from build123d import *

# Parameters (mm, degrees)
SKETCH1_W           = 21
SKETCH1_H           = 30
SKETCH1_R           = 1.75
BOSS_EXTRUDE1_DEPTH = 4
SKETCH2_W           = 21
SKETCH2_H           = 6.5
CUT_EXTRUDE1_DEPTH  = 1
SKETCH3_W           = 1
SKETCH3_H           = 6.5
BOSS_EXTRUDE2_DEPTH = 1
CHAMFER1_SIZE       = 0.5
CHAMFER2_SIZE       = 0.5


with BuildPart() as part:
    # Sketch1 → Boss-Extrude1 (new body)
    with BuildSketch(Plane.XY):
        with Locations((10.5, 15)):
            Rectangle(SKETCH1_W, SKETCH1_H)
        with Locations((4, 4)):
            Circle(SKETCH1_R, mode=Mode.SUBTRACT)
        with Locations((17, 4)):
            Circle(SKETCH1_R, mode=Mode.SUBTRACT)
        with Locations((17, 26)):
            Circle(SKETCH1_R, mode=Mode.SUBTRACT)
        with Locations((4, 26)):
            Circle(SKETCH1_R, mode=Mode.SUBTRACT)
    extrude(amount=BOSS_EXTRUDE1_DEPTH)

    # Sketch2 → Cut-Extrude1 (cut)
    with BuildSketch(Plane.XY.offset(4)):
        with Locations((10.5, 15)):
            Rectangle(SKETCH2_W, SKETCH2_H)
    extrude(amount=-CUT_EXTRUDE1_DEPTH, mode=Mode.SUBTRACT)

    # Sketch3 → Boss-Extrude2 (add)
    with BuildSketch(Plane.XY.offset(3)):
        with Locations((0.5, 15)):
            Rectangle(SKETCH3_W, SKETCH3_H)
        with Locations((2.5, 15)):
            Rectangle(SKETCH3_W, SKETCH3_H)
        with Locations((4.5, 15)):
            Rectangle(SKETCH3_W, SKETCH3_H)
        with Locations((6.5, 15)):
            Rectangle(SKETCH3_W, SKETCH3_H)
        with Locations((8.5, 15)):
            Rectangle(SKETCH3_W, SKETCH3_H)
        with Locations((10.5, 15)):
            Rectangle(SKETCH3_W, SKETCH3_H)
        with Locations((12.5, 15)):
            Rectangle(SKETCH3_W, SKETCH3_H)
        with Locations((14.5, 15)):
            Rectangle(SKETCH3_W, SKETCH3_H)
        with Locations((16.5, 15)):
            Rectangle(SKETCH3_W, SKETCH3_H)
        with Locations((18.5, 15)):
            Rectangle(SKETCH3_W, SKETCH3_H)
        with Locations((20.5, 15)):
            Rectangle(SKETCH3_W, SKETCH3_H)
    extrude(amount=BOSS_EXTRUDE2_DEPTH)

    # Chamfer1
    chamfer1_edges = [part.edges().sort_by_distance(p)[0] for p in [
        (8, 15, 4),
        (9, 15, 4),
        (10, 15, 4),
        (11, 15, 4),
        (12, 15, 4),
        (13, 15, 4),
        (14, 15, 4),
        (15, 15, 4),
        (16, 15, 4),
        (17, 15, 4),
        (18, 15, 4),
        (19, 15, 4),
        (20, 15, 4),
        (1, 15, 4),
        (2, 15, 4),
        (3, 15, 4),
        (4, 15, 4),
        (5, 15, 4),
        (6, 15, 4),
        (7, 15, 4),
    ]]
    chamfer(chamfer1_edges, length=CHAMFER1_SIZE - 0.0001)  # a hair under: the kernel refuses the full size

    # Chamfer2
    chamfer2_edges = [part.edges().sort_by_distance(p)[0] for p in [
        (21, 15, 4),
        (0, 15, 4),
    ]]
    chamfer(chamfer2_edges, length=CHAMFER2_SIZE)


solid = part.part
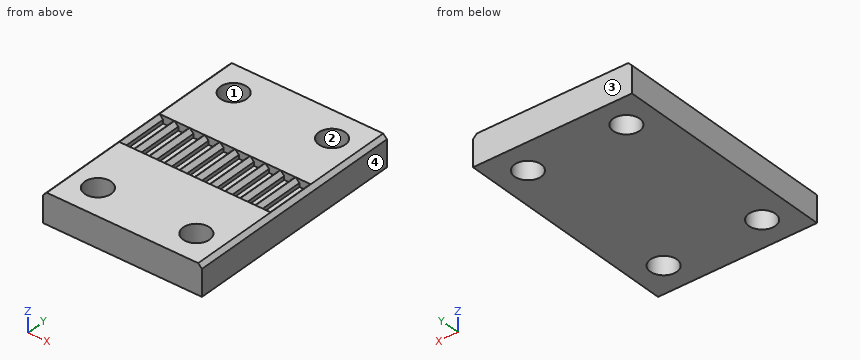
Here's how the part is built. I have some questions about the finished solid (model axes, mm). Face numbers are marked on the shaded views. Round coordinates to 2 decimals unless told otherwise and drop trailing zeros. Order: outer loops, then holes, each group sorted by start corner. A loop starts at its lowest first (then second) coordinate and runs counter-clockwise, first axis right, second up. Notation, with made-up numbers: (3, 87) -> (12, 87) arc R24 ccw to (12, 105) -> close; hole circle Ø2 at (77.25, 88.25). An arc over 180 degrees is marked (long way). Return JSON: item names as keys, results as strings.
Q1. If we section it at B-B on z = 1.8: List the corners of the cut face in (x, y) for me, plus the area to 3 significant figures.
Filled sheet:
{"outline": "(0, 0) -> (21, 0) -> (21, 30) -> (0, 30) -> close; hole circle Ø3.5 at (4, 4); hole circle Ø3.5 at (4, 26); hole circle Ø3.5 at (17, 4); hole circle Ø3.5 at (17, 26)", "area": "592 mm^2"}
Q2. If we section it at A-A on y = 4: List the corners of the cut face in (x, z) for me, plus the area to 4 significant figures.
Filled sheet:
{"outline": "(0, 0) -> (2.25, 0) -> (2.25, 4) -> (0.5, 4) -> (0, 3.5) -> close; (5.75, 0) -> (15.25, 0) -> (15.25, 4) -> (5.75, 4) -> close; (18.75, 0) -> (21, 0) -> (21, 3.5) -> (20.5, 4) -> (18.75, 4) -> close", "area": "55.75 mm^2"}
Q3. For pin 1 Ø0.8 at (x, y) = (19.5, 14) entering from +Z, with a flat end and sliding along its axis, tell me the tip position at first contact or that it passes through.
Filled sheet:
{"pin 1": "stops at z = 3"}
Q4. If we section it at C-C on x = 1.5: List the corners of the cut face in (y, z) for me.
Filled sheet:
{"outline": "(0, 0) -> (30, 0) -> (30, 4) -> (18.25, 4) -> (18.25, 3) -> (11.75, 3) -> (11.75, 4) -> (0, 4) -> close"}
Q5. I need wall thicknesses on line 1 along Y through (x, z) = (4, 0.95); line 2 along X through (y, z) = (25.5, 2.5); line 3 along X through (y, z) = (27.5, 1.55). Which ranges of each line are inside material? Lowest first, please. Write a range as from..to.
Filled sheet:
{"line 1": "y = 0..2.25, 5.75..24.25, 27.75..30", "line 2": "x = 0..2.32, 5.68..15.32, 18.68..21", "line 3": "x = 0..3.1, 4.9..16.1, 17.9..21"}
Q6. If we mould it in two halves opening along Y, with no side actions, what happens to the marked faces 1, 2, 3 and 4? For each: released by +Y, released by -Y, zero draft, split by the parting line, or undercut.
Filled sheet:
{"face 1": "undercut", "face 2": "undercut", "face 3": "released by +Y", "face 4": "zero draft"}
